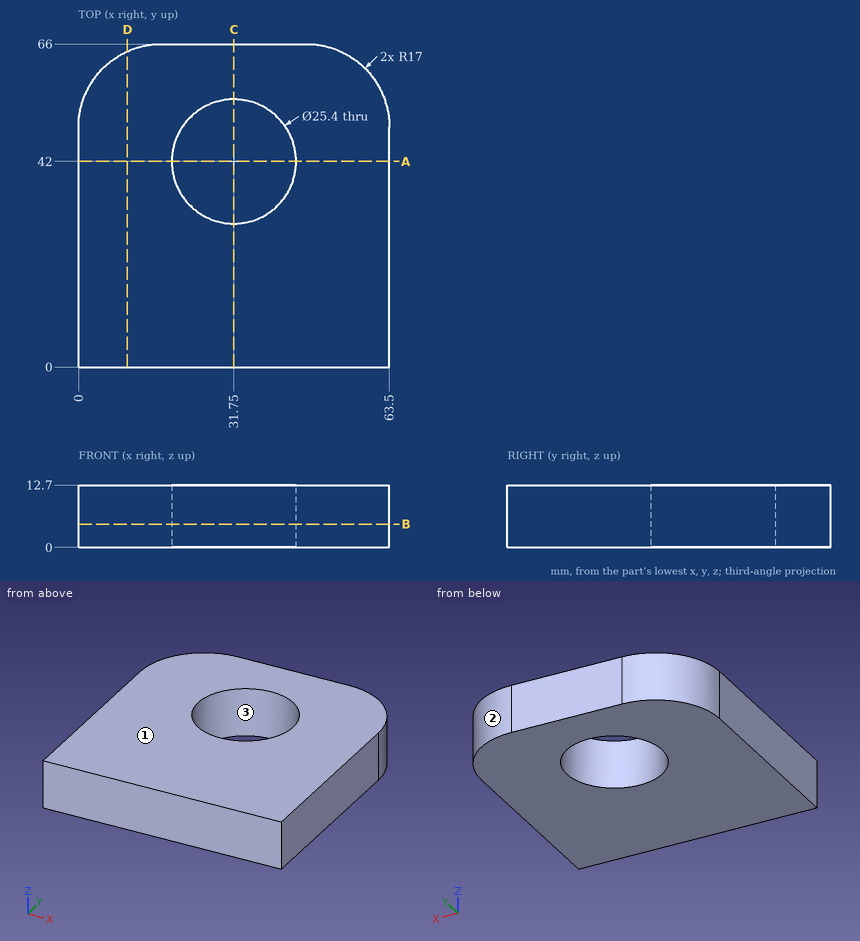
Design review of the part shown in the three views and the two pictorial views. Dimensions are in mm from the part's minimum x, y and z. Round coordinates to 2 decimals unless told otherwise and drop trailing zeros. Order: outer loops, then holes, each group sorted by start corner. A loop starts at its lowest first (then second) coordinate and runs counter-clockwise, first axis right, second up.
Q1. We need section D-D, the plane x = 10. Give the boundary of the cut face in (y, z).
Findings below:
outline: (0, 0) - (64.49, 0) - (64.49, 12.7) - (0, 12.7) - close
Q2. We need section B-B, the plane z = 4.75. Give the boundary of the cut face in (x, y).
Findings below:
outline: (0, 0) - (63.5, 0) - (63.5, 49) arc R17 ccw to (46.5, 66) - (17, 66) arc R17 ccw to (0, 49) - close; hole circle Ø25.4 at (31.75, 42)
Q3. We need section A-A, the plane y = 42. Give the boundary of the cut face in (x, z).
Findings below:
outline: (0, 0) - (19.05, 0) - (19.05, 12.7) - (0, 12.7) - close; (44.45, 0) - (63.5, 0) - (63.5, 12.7) - (44.45, 12.7) - close
Q4. We need section C-C, the plane x = 31.75. Give the boundary of the cut face in (y, z), plus the area to 3 significant figures.
Findings below:
outline: (0, 0) - (29.3, 0) - (29.3, 12.7) - (0, 12.7) - close; (54.7, 0) - (66, 0) - (66, 12.7) - (54.7, 12.7) - close
area: 516 mm2
Q5. Wall thickness on line 1 (Y direction, x = 31.75, z = 3.75); line 2 (X direction, y = 43, z = 5.25); line 3 (Y direction, x = 28, z = 5.25): over which ranges is each line inside the solid? List them lowest first.
Findings below:
line 1: y = 0 to 29.3, 54.7 to 66
line 2: x = 0 to 19.09, 44.41 to 63.5
line 3: y = 0 to 29.87, 54.13 to 66
Q6. Mouldability with a two-part tool opening along X and no side actions: class the marked faces 1, 2 and 3 as pulls with the +X half, pulls with the -X half, needs draft (parallel to the pull), parting line crosses it, or undercut.
Findings below:
face 1: needs draft
face 2: pulls with the +X half
face 3: undercut
